For this review, take the finished solid that the model builds, in its own axes (mm). A direction names the side the tool comes from. Give positions to 0.01 mm unless a question says otherwise; leave off trailing zeros. Write each loop counter-clockwise with the first axis right and the second up, starting at its lowest first coordinate (ties: lowest second). Pieces come first, ordered by that corner, then holes. Notation, with made-up numbers: M -22.5,-3.5 L -0.5,-3.5 A25 cw -0.5,17.5 Z; hole C 89.25,48.25 d4. An arc over 180 degrees is marked long. Answer as a JSON object with one key per item and string values. Group by question number.
```python
from build123d import *

# Parameters (mm, degrees)
SKETCH1_W           = 100
SKETCH1_H           = 100
BOSS_EXTRUDE1_DEPTH = 100
SKETCH2_W           = 87.717538768
SKETCH2_H           = 80.061351375
CUT_EXTRUDE1_DEPTH  = 100
CUT_EXTRUDE2_DEPTH  = 110
SKETCH4_R           = 8.561791054
CUT_EXTRUDE3_DEPTH  = 110


with BuildPart() as part:
    # Sketch1 → Boss-Extrude1 (new body)
    with BuildSketch(Plane(origin=(0, 0, 0), x_dir=(1, 0, 0), z_dir=(0, 1, 0))):
        with Locations((50, 50)):
            Rectangle(SKETCH1_W, SKETCH1_H)
    extrude(amount=BOSS_EXTRUDE1_DEPTH)

    # Sketch2 → Cut-Extrude1 (cut)
    with BuildSketch(Plane(origin=(0, 100, 0), x_dir=(1, 0, 0), z_dir=(0, 1, 0))):
        with Locations((56.141230616, 51.468802688)):
            Rectangle(SKETCH2_W, SKETCH2_H)
    extrude(amount=-CUT_EXTRUDE1_DEPTH, mode=Mode.SUBTRACT)

    # Sketch3 → Cut-Extrude2 (cut)
    with BuildSketch(Plane(origin=(0, 0, -100), x_dir=(-1, 0, 0), z_dir=(0, 0, -1))):
        Polygon((-39.686546089, 44.525018682), (-41.416801354, 57.44192417), (-53.468297277, 62.401931899), (-63.789537935, 54.44503414), (-62.05928267, 41.528128652), (-50.007786746, 36.568120923), align=None)
    extrude(amount=-CUT_EXTRUDE2_DEPTH, mode=Mode.SUBTRACT)

    # Sketch4 → Cut-Extrude3 (cut)
    with BuildSketch(Plane.ZY):
        with Locations((-77.678939526, 55.540564347)):
            Circle(SKETCH4_R)
        with Locations((-22.321060474, 55.540564347)):
            Circle(SKETCH4_R)
    extrude(amount=-CUT_EXTRUDE3_DEPTH, mode=Mode.SUBTRACT)


solid = part.part
```
Item 1: Consider section A-A (x = 14.5). Give the boundary of the cut face in (y, z), plus the area to 3 significant figures.
Item 2: Draft analysis for pull direction X (two halves, no side actions). For faces 1 (the flat face through (12.282, 51, -51)), 2 (the flat face through (38, 49, 0)), 3 (the flat face through (62.937, 48.077, -5.799)), state which applies: released by +X, released by -X, zero draft, split by the parting line, or undercut.
Item 3: Consider section D-D (y = 24.5). Give the boundary of the cut face in (x, z).
Item 4: Consider section C-C (y = 61). Give the boundary of the cut face in (x, z), plus the area to 3 significant figures.
Item 5: Insertion check: P1, Ø10, axis at y = 44.5, z = -68, coming from the +X side; P2, Ø13.5, axis at y = 55.54, z = -22.32, coming from the +X side. Each pin has a flat end and moves straight along its axis. Give the tip position at first contact, or say it passes through.
Item 6: Machinability: for faces 4 (the flat face through (40.54, 50.89, -5.8)), 5 (the flat face through (100, 49, -96)), 6 (the flat face through (65, 51, -91.499)), which of the approach directions +Z, -Z, +X, -X, +Y, -Y give a long, thin tool a straight path to every point of the face, cutting with its end or side? Answer none if there is none.
Item 7: Consider section B-B (z = -16.5). Give the boundary of the cut face in (x, y), plus the area to 3 significant figures.
Item 8: To check wall thickness, follow probe 1 along Z at (x, y) = (23, 51); probe 2 along X at (y, z) = (64, -87); probe 3 along X at (y, z) = (43.5, -9). State the ranges of each line that lie inside material, in increasing order.
Result set:
{
 "1": {"outline": "M 0,-100 L 100,-100 L 100,-91.5 L 0,-91.5 Z; M 0,-11.44 L 100,-11.44 L 100,0 L 0,0 Z", "area": "1,990 mm^2"},
 "2": {"face 1": "released by +X", "face 2": "zero draft", "face 3": "undercut"},
 "3": {"outline": "M 0,-100 L 100,-100 L 100,-91.5 L 12.28,-91.5 L 12.28,-11.44 L 100,-11.44 L 100,0 L 0,0 Z"},
 "4": {"outline": "M 0,-100 L 50.06,-100 L 50.06,-91.5 L 12.28,-91.5 L 12.28,-84.27 L 0,-84.27 Z; M 0,-71.08 L 12.28,-71.08 L 12.28,-28.92 L 0,-28.92 Z; M 0,-15.73 L 12.28,-15.73 L 12.28,-11.44 L 50.06,-11.44 L 50.06,0 L 0,0 Z; M 55.29,-100 L 100,-100 L 100,-91.5 L 55.29,-91.5 Z; M 55.29,-11.44 L 100,-11.44 L 100,0 L 55.29,0 Z", "area": "2,550 mm^2"},
 "5": {"P1": "stops at x = 12.28", "P2": "passes through"},
 "6": {"face 4": "+Z, -Z", "face 5": "+Z, -Z, +X, +Y, -Y", "face 6": "+X, +Y, -Y"},
 "7": {"outline": "M 0,0 L 12.28,0 L 12.28,49.26 L 0,49.26 Z; M 0,61.82 L 12.28,61.82 L 12.28,100 L 0,100 Z", "area": "1,070 mm^2"},
 "8": {"probe 1": "z = -100 to -91.5, -11.44 to 0", "probe 2": "x = 0 to 12.28", "probe 3": "x = 0 to 41.02, 62.32 to 100"}
}
